```python
from build123d import *

# Parameters (mm, degrees)
F0_R     = 23.8231892188
F0_R_2   = 16.1761148504
F0_R_3   = 1.4754891284
F1_DEPTH = 25.4


with BuildPart() as f1:
    # F0 (on Front) → F1 (new body)
    with BuildSketch(Plane.XZ):
        with BuildLine():
            ThreePointArc((59.4117882899, 54.835062474), (30.0941746682, 72.4310516269), (0.7765610465, 54.835062474))
            Line((0.7765610465, 54.835062474), (59.4117882899, 54.835062474))
        make_face()
        with BuildLine():
            Line((59.4117882899, 54.835062474), (0.7765610465, 54.835062474))
            ThreePointArc((0.7765610465, 54.835062474), (22.0410833069, 6.9782518983), (63.3159871103, 39.2092391849))
            ThreePointArc((63.3159871103, 39.2092391849), (62.3251619547, 47.2623305461), (59.4117882899, 54.835062474))
        make_face()
        with BuildLine():
            Line((-19.0199100919, 54.835062474), (-67.2114855104, 54.835062474))
            ThreePointArc((-67.2114855104, 54.835062474), (-71.7847333832, 46.8469948963), (-73.788613081, 37.8632158535))
            Line((-73.788613081, 37.8632158535), (-73.788613081, 33.6104571325))
            ThreePointArc((-73.788613081, 33.6104571325), (-42.0518711488, 5.0087142952), (-12.3691659487, 35.736836493))
            ThreePointArc((-12.3691659487, 35.736836493), (-14.079417691, 45.8483971203), (-19.0199100919, 54.835062474))
        make_face()
        with BuildLine():
            ThreePointArc((-19.0199100919, 54.835062474), (-43.1156978011, 66.4833683454), (-67.2114855104, 54.835062474))
            Line((-67.2114855104, 54.835062474), (-19.0199100919, 54.835062474))
        make_face()
        with BuildLine():
            Line((0.7765610465, 54.835062474), (-19.0199100919, 54.835062474))
            ThreePointArc((-19.0199100919, 54.835062474), (-14.079417691, 45.8483971203), (-12.3691659487, 35.736836493))
            ThreePointArc((-12.3691659487, 35.736836493), (-42.0518711488, 5.0087142952), (-73.788613081, 33.6104571325))
            Line((-73.788613081, 33.6104571325), (-73.788613081, -50.20519346))
            Line((-73.788613081, -50.20519346), (74.6567100286, -50.20519346))
            Line((74.6567100286, -50.20519346), (74.6567100286, 54.835062474))
            Line((74.6567100286, 54.835062474), (59.4117882899, 54.835062474))
            ThreePointArc((59.4117882899, 54.835062474), (62.3251619547, 47.2623305461), (63.3159871103, 39.2092391849))
            ThreePointArc((63.3159871103, 39.2092391849), (22.0410833069, 6.9782518983), (0.7765610465, 54.835062474))
        make_face()
        with Locations((-38.775190711, -19.2429125309)):
            Circle(F0_R, mode=Mode.SUBTRACT)
        with Locations((32.119743526, -15.7705061138)):
            Circle(F0_R_2, mode=Mode.SUBTRACT)
        with Locations((32.119743526, -15.7705061138)):
            Circle(F0_R_2)
        with Locations((32.119743526, -15.7705061138)):
            Circle(F0_R_3, mode=Mode.SUBTRACT)
    extrude(amount=F1_DEPTH)


solid = f1.part
```
Source: CAD feature listing. Evaluate the final solid. Frame: model axes, mm. A direction names the side the tool comes from. Round coordinates to 2 decimals unless told otherwise and drop trailing zeros. Loops run counter-clockwise (first coordinate to the right, second up) from the corner with the lowest first, then second, coordinate; pieces in that order, holes last. Notation, with made-up numbers: M 69.5,29 L 91.5,29 A4 ccw 91.5,34 Z; hole C -4,7 d6. An arc over 180 degrees is marked long. Use a Markdown table: item, result. Add a question column.
1. Section query D-D on x = 49.5. Return the cut outline in (y, z), then the cut area to 3 significant figures.
2. Mould query, pull axis X, two halves, no side actions, for faces 1 (the cylindrical face through (31.928, -12.522, -14.308)), 2 (the flat face through (-73.789, -13, -6)), 3 (the flat face through (74.657, -13, 2)). Classes: pulls with the +X half, pulls with the -X half, needs draft (parallel to the pull), parting line crosses it, or undercut.
3. Contact query for flat-ended pins moving along their axis: P1, Ø8, axis at x = -36, z = 49, coming from the +Y side; P2, Ø6, axis at x = -12.5, y = -10, coming from the +Z side; P3, Ø10, axis at x = 5, y = -6, coming from the +Z side. Output: stop coordinate, or through.
4. Line query: line 1 (Z direction, x = 64, y = -10); line 2 (Z direction, x = -34.5, y = -1); line 3 (X direction, y = -15, z = -36.5). Output: solid intervals per line, ascending.
5. Reachability of faces 4 (the flat face through (-1, -13, -50.205)), 5 (the flat face through (67, -13, 54.835)), 6 (the flat face through (-9, -13, 54.835)) from +Z, -Z, +X, -X, +Y, -Y: full face, straight path, thin tool, end or side. Return the list, or none.
6. Section query C-C on y = -2.75. Return the cut outline in (x, z).
7. Section query A-A on x = -40. Return the cut outline in (y, z).
8. Section query B-B on z = -5. Return the cut outline in (x, y).
Reported:
| question | item | result |
|---|---|---|
| 1 | outline | M -25.4,-50.21 L 0,-50.21 L 0,66.17 L -25.4,66.17 Z |
| 1 | area | 2,960 mm² |
| 2 | face 1 | undercut |
| 2 | face 2 | pulls with the -X half |
| 2 | face 3 | pulls with the +X half |
| 3 | P1 | stops at y = 0 |
| 3 | P2 | stops at z = 54.84 |
| 3 | P3 | stops at z = 65.67 |
| 4 | line 1 | z = -50.21 to 54.84 |
| 4 | line 2 | z = -50.21 to -42.68, 4.19 to 65.25 |
| 4 | line 3 | x = -73.79 to -55.2, -22.35 to 74.66 |
| 5 | face 4 | -Z, +X, -X, +Y, -Y |
| 5 | face 5 | +Z, +X, +Y, -Y |
| 5 | face 6 | +Z, +Y, -Y |
| 6 | outline | M -73.79,-50.21 L 74.66,-50.21 L 74.66,54.84 L 59.41,54.84 A33.22 ccw 0.78,54.84 L -19.02,54.84 A30.75 ccw -73.79,37.86 Z; hole C -38.78,-19.24 d47.65; hole C 32.12,-15.77 d2.95 |
| 7 | outline | M -25.4,-50.21 L 0,-50.21 L 0,-43.03 L -25.4,-43.03 Z; M -25.4,4.55 L 0,4.55 L 0,66.33 L -25.4,66.33 Z |
| 8 | outline | M -73.79,-25.4 L -57.87,-25.4 L -57.87,0 L -73.79,0 Z; M -19.68,-25.4 L 74.66,-25.4 L 74.66,0 L -19.68,0 Z |
